```python
from build123d import *

# Parameters (mm, degrees)
SKETCH_1_W               = 90
SKETCH_1_H               = 48
EXTRUDE_1_DEPTH          = 8
SKETCH_6_R               = 1.8
CUT_EXTRUDE_4_DEPTH      = 3
MIRROR_6_COPY_1_SKETCH_R = 1.8
MIRROR_6_COPY_1_DEPTH    = 3
SKETCH_7_W               = 16
SKETCH_7_H               = 15
CUT_EXTRUDE_5_DEPTH      = 2.5
SKETCH_4_R               = 2
CUT_EXTRUDE_6_DEPTH      = 10
PATTERN_CIRCULAR_1_COUNT = 3


with BuildPart() as part:
    # 草图1 → 凸台-拉伸1 (new body)
    with BuildSketch(Plane.XY):
        Rectangle(SKETCH_1_W, SKETCH_1_H)
    extrude(amount=EXTRUDE_1_DEPTH)

    # 草图6 → 切除-拉伸4 (cut)
    with BuildSketch(Plane(origin=(0, 0, 0), x_dir=(-1, 0, 0), z_dir=(0, 0, -1))):
        with Locations((-41, 21)):
            Circle(SKETCH_6_R)
    cut_extrude_4 = extrude(amount=-CUT_EXTRUDE_4_DEPTH, mode=Mode.SUBTRACT)

    # 镜向5: 切除-拉伸4 across plane
    add(cut_extrude_4.mirror(Plane.ZX), mode=Mode.SUBTRACT)

    # 镜向6: 切除-拉伸4 across plane
    add(cut_extrude_4.mirror(Plane(origin=(0, 0, 0), x_dir=(0, 0, 1), z_dir=(1, 0, 0))), mode=Mode.SUBTRACT)

    # 镜向6 copy 1 sketch → 镜向6 copy 1 (cut)
    with BuildSketch(Plane(origin=(0, 0, 0), x_dir=(1, 0, 0), z_dir=(0, 0, -1))):
        with Locations((-41, 21)):
            Circle(MIRROR_6_COPY_1_SKETCH_R)
    extrude(amount=-MIRROR_6_COPY_1_DEPTH, mode=Mode.SUBTRACT)

    # 草图7 → 切除-拉伸5 (cut)
    with BuildSketch(Plane(origin=(0, 0, 0), x_dir=(-1, 0, 0), z_dir=(0, 0, -1))):
        with Locations((-45.051826461, 0)):
            Rectangle(SKETCH_7_W, SKETCH_7_H)
    cut_extrude_5 = extrude(amount=-CUT_EXTRUDE_5_DEPTH, mode=Mode.SUBTRACT)

    # 镜向7: 切除-拉伸5 across plane
    add(cut_extrude_5.mirror(Plane(origin=(0, 0, 0), x_dir=(0, 0, 1), z_dir=(1, 0, 0))), mode=Mode.SUBTRACT)

    # 草图4 → 切除-拉伸6 (cut)
    with BuildSketch(Plane.XY.offset(8)):
        with Locations((0, 8.85)):
            Circle(SKETCH_4_R)
    cut_extrude_6 = extrude(amount=-CUT_EXTRUDE_6_DEPTH, mode=Mode.SUBTRACT)

    # 阵列(圆周)1: 切除-拉伸6 ×3 about axis
    pattern_circular_1_axis = Axis((0, -0.027607952, 0), (0, 0, 1))
    for i in range(1, PATTERN_CIRCULAR_1_COUNT):
        add(cut_extrude_6.rotate(pattern_circular_1_axis, i * 360 / PATTERN_CIRCULAR_1_COUNT), mode=Mode.SUBTRACT)


solid = part.part
```
Here's how the part is built. I have some questions about the finished solid (model axes, mm). A direction names the side the tool comes from. Coordinates: 2 decimals unless noted, no trailing zeros. Loops run counter-clockwise (first coordinate to the right, second up) from the corner with the lowest first, then second, coordinate; pieces in that order, holes last. Notation, with made-up numbers: M 83.5,-1 L 141.5,-1 A27 cw 141.5,25 Z; hole C 79,3 d6. An arc over 180 degrees is marked long. One line per item, written item: value.
1. On a 3-axis mill with a long thin cutter (end or side, diameter ignored), from which of +Z, -Z, +X, -X, +Y, -Y can I reach the whole of each face in a straight line? I mean faces 5 (the cylindrical face through (-40.032, -22.518, 1.479)), 6 (the flat face through (-1, -24, 4)), 7 (the flat face through (41, 0, 2.5)), 8 (the flat face through (-41, 7.5, 1)). Say none if no direction works.
Geometry says:
face 5: -Z
face 6: +Z, -Z, +X, -X, -Y
face 7: -Z, +X
face 8: -Z, -X
2. Imagine slicing it at A-A (y = 8.85). List the corners of the cut face in (x, z) for me.
Geometry says:
outline: M -45,0 L -2,0 L -2,8 L -45,8 Z; M 2,0 L 45,0 L 45,8 L 2,8 Z
3. Imagine slicing it at D-D (z = 1.5). List the corners of the cut face in (x, y) for me, and give its area (3 significant figures).
Geometry says:
outline: M -45,-24 L 45,-24 L 45,-7.5 L 37.05,-7.5 L 37.05,7.5 L 45,7.5 L 45,24 L -45,24 L -45,7.5 L -37.05,7.5 L -37.05,-7.5 L -45,-7.5 Z; hole C -41,-21 d3.6; hole C -41,21 d3.6; hole C -7.69,-4.47 d4; hole C 0,8.85 d4; hole C 7.69,-4.47 d4; hole C 41,-21 d3.6; hole C 41,21 d3.6
area: 4,000 mm2
4. Will these pins go through, and if not, where does the flat tip stop? pin 1 Ø2.5 at (x, y) = (42, -1.5) entering from -Z; pin 2 Ø1.1 at (x, y) = (-40.5, 20.5) entering from -Z.
Geometry says:
pin 1: stops at z = 2.5
pin 2: stops at z = 3
5. Imagine slicing it at C-C (y = -21). List the corners of the cut face in (x, z) for me.
Geometry says:
outline: M -45,0 L -42.8,0 L -42.8,3 L -39.2,3 L -39.2,0 L 39.2,0 L 39.2,3 L 42.8,3 L 42.8,0 L 45,0 L 45,8 L -45,8 Z
6. Thinking about a two-plate mould opening in X: for faces 1 (the flat face through (-45, 0, 4)), 2 (the flat face through (45, 0, 4)), 3 (the flat face through (-41, -7.5, 1)), 4 (the cylindrical face through (-9.686, -4.378, 4.056)), which applies, +X half, -X half, draft (parallel to the pull), parting line (faces both ways), or undercut?
Geometry says:
face 1: -X half
face 2: +X half
face 3: draft
face 4: undercut
7. Please list where these lines run through material, in increasing order: probe 1 along Y at (x, z) = (41, 0.75); probe 2 along X at (y, z) = (-21, 1.5); probe 3 along Y at (x, z) = (0, 3).
Geometry says:
probe 1: y = -24 to -22.8, -19.2 to -7.5, 7.5 to 19.2, 22.8 to 24
probe 2: x = -45 to -42.8, -39.2 to 39.2, 42.8 to 45
probe 3: y = -24 to 6.85, 10.85 to 24
8. Imagine slicing it at B-B (x = 41). List the corners of the cut face in (y, z) for me, and give its area (3 significant figures).
Geometry says:
outline: M -24,0 L -22.8,0 L -22.8,3 L -19.2,3 L -19.2,0 L -7.5,0 L -7.5,2.5 L 7.5,2.5 L 7.5,0 L 19.2,0 L 19.2,3 L 22.8,3 L 22.8,0 L 24,0 L 24,8 L -24,8 Z
area: 325 mm2
